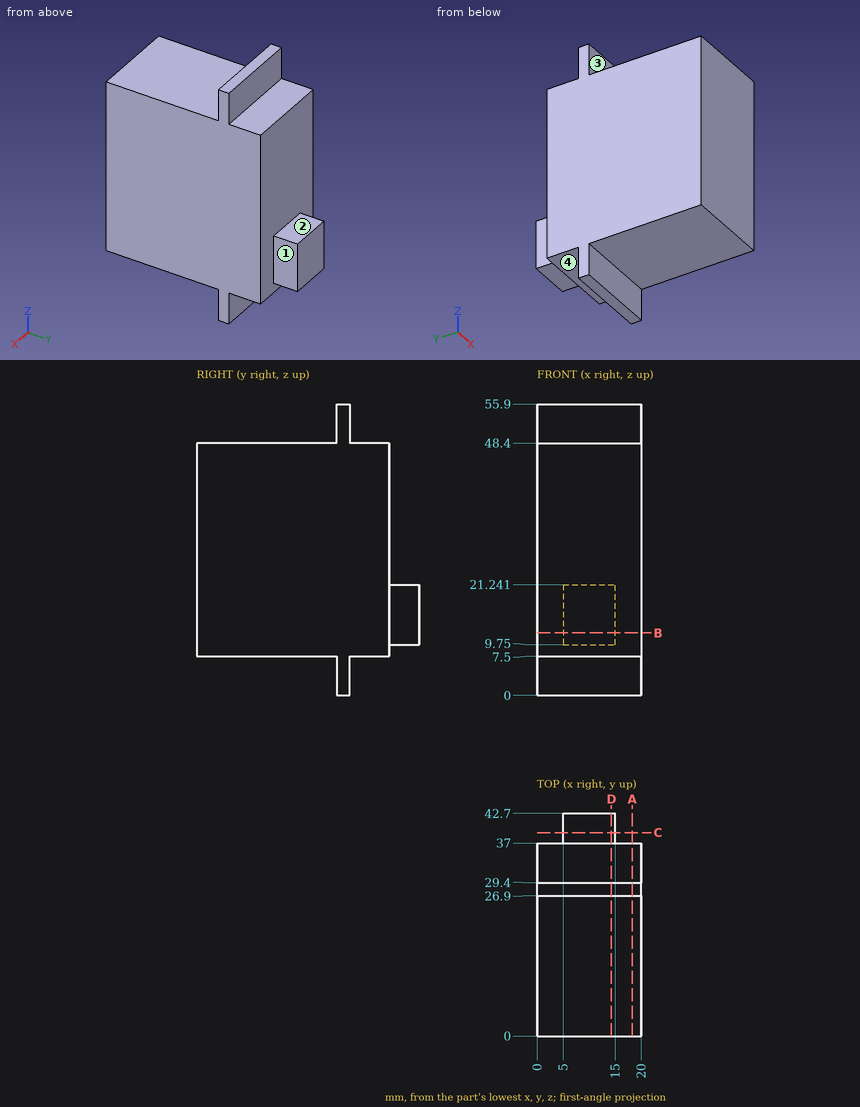
Design review of the part shown in the three views and the two pictorial views. Dimensions are in mm from the part's minimum x, y and z. A direction names the side the tool comes from. Coordinates: 2 decimals unless noted, no trailing zeros. Order: outer loops, then holes, each group sorted by start corner. A loop starts at its lowest first (then second) coordinate and runs counter-clockwise, first axis right, second up. Notation, with made-up numbers: (-24, 21.25) -> (-5, 21.25) arc R32 ccw to (-5, 55.25) -> close; hole circle Ø11 at (-0.5, -20). An arc over 180 degrees is marked (long way). Use one line per item in the form item = value. Start each with the question number.
(1) Add section D-D on x = 14.25. State the section outline as (y, z) points.
(2) Add section B-B on z = 12. State the section outline as (x, y) points, plus the area to 3 significant figures.
(3) For probe 1 along Z at (x, y) = (15.5, 20.5); probe 2 along Y at (x, z) = (10, 51.5); probe 3 along Y at (x, z) = (10.25, 38), list the stretches that pass through material, from the lowest coordinate up.
(4) Insertion check: pin 1 (6 mm diameter, centred on x = 9.5, y = 34, fed in from -Z); pin 2 (8 mm diameter, centred on x = 13, z = 52.5, fed in from -Y); pin 3 (1.5 mm diameter, centred on y = 11.5, z = 49, fed in from +X); pin 4 (10 mm diameter, centred on x = 12.5, z = 28, fed in from +Y). Each pin has a flat end and moves straight along its axis. Give the tip position at first contact, or say it passes through.
(5) For the marked faces 1, 2, 3 and 4, list the 3-axis set-ups (+Z, -Z, +X, -X, +Y, -Y) from which the entire face can be reached by the end or side of a thin tool; tool diameter is ignored.
(6) Add section A-A on x = 18.25. State the section outline as (y, z) points, plus the area to 3 significant figures.
(7) Add section C-C on y = 39. State the section outline as (x, z) points, plus the area to 3 significant figures.
Answer block:
q1.outline = (0, 7.5) -> (26.9, 7.5) -> (26.9, 0) -> (29.4, 0) -> (29.4, 7.5) -> (37, 7.5) -> (37, 9.75) -> (42.7, 9.75) -> (42.7, 21.24) -> (37, 21.24) -> (37, 48.4) -> (29.4, 48.4) -> (29.4, 55.9) -> (26.9, 55.9) -> (26.9, 48.4) -> (0, 48.4) -> close
q2.outline = (0, 0) -> (20, 0) -> (20, 37) -> (15, 37) -> (15, 42.7) -> (5, 42.7) -> (5, 37) -> (0, 37) -> close
q2.area = 797 mm²
q3.probe_1 = 7.5 to 48.4
q3.probe_2 = 26.9 to 29.4
q3.probe_3 = 0 to 37
q4.pin_1 = 7.5
q4.pin_2 = 26.9
q4.pin_3 = 20
q4.pin_4 = 37
q5.face_1 = +Z, -Z, +X, +Y
q5.face_2 = +Z, +X, -X, +Y
q5.face_3 = +Z, +X, -X, -Y
q5.face_4 = -Z, +X, -X, +Y
q6.outline = (0, 7.5) -> (26.9, 7.5) -> (26.9, 0) -> (29.4, 0) -> (29.4, 7.5) -> (37, 7.5) -> (37, 48.4) -> (29.4, 48.4) -> (29.4, 55.9) -> (26.9, 55.9) -> (26.9, 48.4) -> (0, 48.4) -> close
q6.area = 1,550 mm²
q7.outline = (5, 9.75) -> (15, 9.75) -> (15, 21.24) -> (5, 21.24) -> close
q7.area = 115 mm²
